Model file for the job. Use its own axes, mm. Face numbers are marked on the shaded views. A direction names the side the tool comes from. Coordinates: 2 decimals unless noted, no trailing zeros. Order: outer loops, then holes, each group sorted by start corner. A loop starts at its lowest first (then second) coordinate and runs counter-clockwise, first axis right, second up.
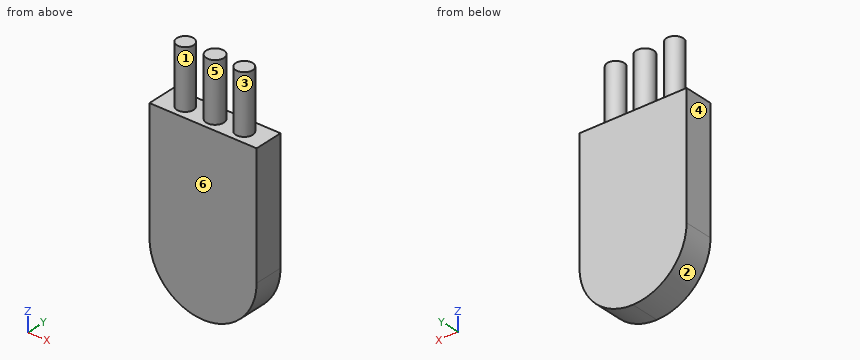
Autodesk Inventor part; units mm, degrees
ref_plane "YZ Plane" through (0, 0, 0) normal (1, 0, 0) x (0, 1, 0)
ref_plane "XZ Plane" through (0, 0, 0) normal (0, 1, 0) x (-1, 0, 0)
ref_plane "XY Plane" through (0, 0, 0) normal (0, 0, 1) x (1, 0, 0)
sketch "Sketch1" plane through (0, 0, 0) normal (0, 1, 0) x (-1, 0, 0)
  line L0 (0, 0) -> (55, 0)
  line L1 (55, 0) -> (55, -90)
  line L2 (55, -90) -> (0, -90)
  line L3 (0, -90) -> (0, 0)
  dimension "d0" = 90
  dimension "d1" = 55
extrude "Extrusion1" add sketch "Sketch1" along normal blind 15
full round fillet "Fillet1" first side at (0, 5, -30) centre faces at (-18.3333, 5, -90) second side at (-55, 5, -60)
sketch "Sketch2" plane through (-55, 0, 0) normal (0, 0, 1) x (1, 0, 0)
  circle A0 centre (12.5986, 7.0416) radius 4.3081
  circle A1 centre (27.8976, 7.0416) radius 4.5356
  circle A2 centre (42.8926, 7.0416) radius 4.3708
  point P0 (55, 0)
extrude "Extrusion2" add sketch "Sketch2" along normal blind 30
sketch "Sketch3" plane through (0, 15, 0) normal (0, 1, 0) x (1, 0, 0)
  line L0 (-48.594, 65.8616) -> (-7.6272, 65.8616) construction
  line L1 (-7.6272, 65.8616) -> (-7.6272, 56.4823) construction
  line L2 (-7.6272, 56.4823) -> (-48.594, 56.4823) construction
  line L3 (-48.594, 56.4823) -> (-48.594, 65.8616) construction
  point P0 (0, 0)
  dimension "d2" = 15
  dimension "d3" = 0
properties part number "tmp 36 now"
Q1. Probe line 1 (X direction, y = 4.25, z = 12); line 2 (X direction, y = 6.5, z = 21); line 3 (Z direction, x = -21.5, y = 1). List the from-to ranges inside material, lowest first.
Established:
line 1: x = -45.68 to -39.12, -30.68 to -23.53, -15.47 to -8.74
line 2: x = -46.68 to -38.13, -31.61 to -22.6, -16.44 to -7.77
line 3: z = -89.34 to 0
Q2. Cut at C-C, the plane z = -78. List the corners of the cut face in (x, y), plus the area to 3 significant figures.
Established:
outline: (-50.22, 0) - (-4.78, 0) - (-4.78, 15) - (-50.22, 15) - close
area: 681 mm2
Q3. Drop flat-ended pins along their axis: P1, Ø2, axis at x = -12, y = 9, coming from the -Z side; P2, Ø5, axis at x = -6, y = 10.5, coming from the -Z side; P3, Ø4, axis at x = -13, y = 11, coming from the -Z side. Give the stop position or say it passes through.
Established:
P1: stops at z = -85.87
P2: stops at z = -82.38
P3: stops at z = -86.99
Q4. Mould opens along X. For the marked faces 3, 4, 5 and 6 say: pulls with the +X half, pulls with the -X half, needs draft (parallel to the pull), parting line crosses it, or undercut.
Established:
face 3: undercut
face 4: pulls with the -X half
face 5: undercut
face 6: needs draft
Q5. Which spindle directions (+Z, -Z, +X, -X, +Y, -Y) get a long thin tool onto all of the face, cutting with end or side? Do the marked faces 1 and 2. Say none if no direction does.
Established:
face 1: +Z
face 2: -Z, -X, +Y, -Y
Q6. Cut at B-B, the plane x = -40. List the corners of the cut face in (y, z).
Established:
outline: (0, -86.99) - (15, -86.99) - (15, 0) - (10.62, 0) - (10.62, 30) - (3.46, 30) - (3.46, 0) - (0, 0) - close
